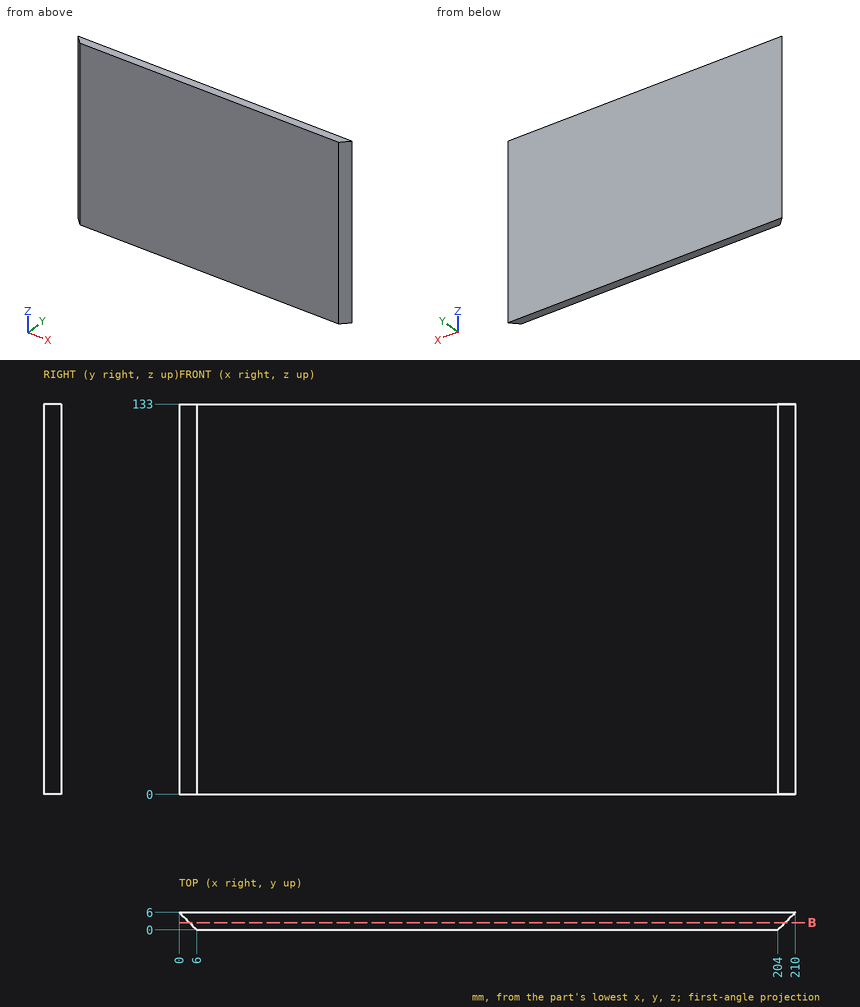
The figure shows three views and two pictorial views of one solid part (mm, origin at its lowest corner). Answer the questions. Give positions to 0.01 mm unless a question says otherwise; leave off trailing zeros. Loops run counter-clockwise (first coordinate to the right, second up) from the corner with the lowest first, then second, coordinate; pieces in that order, holes last. Notation, with made-up numbers: (37.25, -3) - (43.25, -3) arc R18 ccw to (43.25, 14) - close; hole circle Ø11 at (79.5, 30.25). An arc over 180 degrees is marked (long way). Use one line per item in the form item = value.
1. Section B-B on y = 2.5 is taken. Give the vertices of the cut face in (x, z), then the cut area to 3 significant figures.
Calculated:
outline = (3.5, 0) - (206.5, 0) - (206.5, 133) - (3.5, 133) - close
area = 27,000 mm^2
2. Find the intervals of material crossed by line 1 along X through (y, z) = (2.5, 53.5); line 2 along X through (y, z) = (5.75, 78), in increasing order. Write a range as [from, to].
Calculated:
line_1 = [3.5, 206.5]
line_2 = [0.25, 209.75]
3. Given pin 1 Ø1.5 at (y, z) = (3.5, 46) entering from +X; pin 2 Ø1 at (x, y) = (150.5, 3.5) entering from -Z; pin 3 Ø3 at (y, z) = (1.5, 39) entering from +X, each flat-ended and moving along its own axis, determine where each tip first touches the part or whether it passes through.
Calculated:
pin_1 = 208.25
pin_2 = 0
pin_3 = 207
